```python
from build123d import *

# Parameters (mm, degrees)
SKETCH_1_R      = 25
SKETCH_1_R_2    = 2.1
EXTRUDE_1_DEPTH = 5
SKETCH_2_R      = 25
SKETCH_2_R_2    = 24
SKETCH_2_R_3    = 12
EXTRUDE_2_DEPTH = 4
FILLET_1_R      = 1
SKETCH_3_R      = 8
EXTRUDE_3_DEPTH = 15


with BuildPart() as part:
    # Эскиз1 → Бобышка-Вытянуть1 (new body)
    with BuildSketch(Plane(origin=(0, 0, 0), x_dir=(1, 0, 0), z_dir=(0, 1, 0))):
        with Locations(Location((0, 0, 0), (0, 0, 270))):
            Circle(SKETCH_1_R)
        with Locations(Location((-18, 0, 0), (0, 0, 270))):
            Circle(SKETCH_1_R_2, mode=Mode.SUBTRACT)
        with Locations(Location((-12.727922061, 12.727922061, 0), (0, 0, 270))):
            Circle(SKETCH_1_R_2, mode=Mode.SUBTRACT)
        with Locations(Location((0, 18, 0), (0, 0, 270))):
            Circle(SKETCH_1_R_2, mode=Mode.SUBTRACT)
        with Locations(Location((12.727922061, 12.727922061, 0), (0, 0, 270))):
            Circle(SKETCH_1_R_2, mode=Mode.SUBTRACT)
        with Locations(Location((18, 0, 0), (0, 0, 270))):
            Circle(SKETCH_1_R_2, mode=Mode.SUBTRACT)
        with Locations(Location((12.727922061, -12.727922061, 0), (0, 0, 270))):
            Circle(SKETCH_1_R_2, mode=Mode.SUBTRACT)
        with Locations(Location((0, -18, 0), (0, 0, 270))):
            Circle(SKETCH_1_R_2, mode=Mode.SUBTRACT)
        with Locations(Location((-12.727922061, -12.727922061, 0), (0, 0, 270))):
            Circle(SKETCH_1_R_2, mode=Mode.SUBTRACT)
    extrude(amount=EXTRUDE_1_DEPTH)

    # Эскиз2 → Бобышка-Вытянуть2 (add)
    # profile 1 of 10: a face of its own
    with BuildSketch(Plane(origin=(0, 5, 0), x_dir=(1, 0, 0), z_dir=(0, 1, 0))):
        with Locations(Location((0, 0, 0), (0, 0, 270))):
            Circle(SKETCH_2_R)
        Circle(SKETCH_2_R_2, mode=Mode.SUBTRACT)
    # profile 2 of 10: a face of its own
    with BuildSketch(Plane(origin=(0, 5, 0), x_dir=(1, 0, 0), z_dir=(0, 1, 0))):
        Circle(SKETCH_2_R_3)
    # profile 3 of 10: a face of its own
    with BuildSketch(Plane(origin=(0, 5, 0), x_dir=(1, 0, 0), z_dir=(0, 1, 0))):
        with BuildLine():
            Line((-10.332266323, 21.662046824), (-5.166133162, 10.831023412))
            ThreePointArc((-5.166133162, 10.831023412), (-4.592201188, 11.08655439), (-4.005682311, 11.311697893))
            Line((-4.005682311, 11.311697893), (-8.011364622, 22.623395786))
            ThreePointArc((-8.011364622, 22.623395786), (-9.184402377, 22.17310878), (-10.332266323, 21.662046824))
        make_face()
    # profile 4 of 10: a face of its own
    with BuildSketch(Plane(origin=(0, 5, 0), x_dir=(1, 0, 0), z_dir=(0, 1, 0))):
        with BuildLine():
            Line((8.011364622, 22.623395786), (4.005682311, 11.311697893))
            ThreePointArc((4.005682311, 11.311697893), (4.592201188, 11.08655439), (5.166133162, 10.831023412))
            Line((5.166133162, 10.831023412), (10.332266323, 21.662046824))
            ThreePointArc((10.332266323, 21.662046824), (9.184402377, 22.17310878), (8.011364622, 22.623395786))
        make_face()
    # profile 5 of 10: a face of its own
    with BuildSketch(Plane(origin=(0, 5, 0), x_dir=(1, 0, 0), z_dir=(0, 1, 0))):
        with BuildLine():
            ThreePointArc((10.831023412, 5.166133162), (11.08655439, 4.592201188), (11.311697893, 4.005682311))
            Line((11.311697893, 4.005682311), (22.623395786, 8.011364622))
            ThreePointArc((22.623395786, 8.011364622), (22.17310878, 9.184402377), (21.662046824, 10.332266323))
            Line((21.662046824, 10.332266323), (10.831023412, 5.166133162))
        make_face()
    # profile 6 of 10: a face of its own
    with BuildSketch(Plane(origin=(0, 5, 0), x_dir=(1, 0, 0), z_dir=(0, 1, 0))):
        with BuildLine():
            ThreePointArc((11.311697893, -4.005682311), (11.08655439, -4.592201188), (10.831023412, -5.166133162))
            Line((10.831023412, -5.166133162), (21.662046824, -10.332266323))
            ThreePointArc((21.662046824, -10.332266323), (22.17310878, -9.184402377), (22.623395786, -8.011364622))
            Line((22.623395786, -8.011364622), (11.311697893, -4.005682311))
        make_face()
    # profile 7 of 10: a face of its own
    with BuildSketch(Plane(origin=(0, 5, 0), x_dir=(1, 0, 0), z_dir=(0, 1, 0))):
        with BuildLine():
            ThreePointArc((5.166133162, -10.831023412), (4.592201188, -11.08655439), (4.005682311, -11.311697893))
            Line((4.005682311, -11.311697893), (8.011364622, -22.623395786))
            ThreePointArc((8.011364622, -22.623395786), (9.184402377, -22.17310878), (10.332266323, -21.662046824))
            Line((10.332266323, -21.662046824), (5.166133162, -10.831023412))
        make_face()
    # profile 8 of 10: a face of its own
    with BuildSketch(Plane(origin=(0, 5, 0), x_dir=(1, 0, 0), z_dir=(0, 1, 0))):
        with BuildLine():
            ThreePointArc((-4.005682311, -11.311697893), (-4.592201188, -11.08655439), (-5.166133162, -10.831023412))
            Line((-5.166133162, -10.831023412), (-10.332266323, -21.662046824))
            ThreePointArc((-10.332266323, -21.662046824), (-9.184402377, -22.17310878), (-8.011364622, -22.623395786))
            Line((-8.011364622, -22.623395786), (-4.005682311, -11.311697893))
        make_face()
    # profile 9 of 10: a face of its own
    with BuildSketch(Plane(origin=(0, 5, 0), x_dir=(1, 0, 0), z_dir=(0, 1, 0))):
        with BuildLine():
            Line((-21.662046824, -10.332266323), (-10.831023412, -5.166133162))
            ThreePointArc((-10.831023412, -5.166133162), (-11.08655439, -4.592201188), (-11.311697893, -4.005682311))
            Line((-11.311697893, -4.005682311), (-22.623395786, -8.011364622))
            ThreePointArc((-22.623395786, -8.011364622), (-22.17310878, -9.184402377), (-21.662046824, -10.332266323))
        make_face()
    # profile 10 of 10: a face of its own
    with BuildSketch(Plane(origin=(0, 5, 0), x_dir=(1, 0, 0), z_dir=(0, 1, 0))):
        with BuildLine():
            Line((-22.623395786, 8.011364622), (-11.311697893, 4.005682311))
            ThreePointArc((-11.311697893, 4.005682311), (-11.08655439, 4.592201188), (-10.831023412, 5.166133162))
            Line((-10.831023412, 5.166133162), (-21.662046824, 10.332266323))
            ThreePointArc((-21.662046824, 10.332266323), (-22.17310878, 9.184402377), (-22.623395786, 8.011364622))
        make_face()
    extrude(amount=EXTRUDE_2_DEPTH)

    # Скругление1
    fillet_1_edges = [part.edges().sort_by_distance(p)[0] for p in [
        (5.166133162, 7, 10.831023412),
        (10.831023412, 7, 5.166133162),
        (21.662046824, 7, 10.332266323),
        (22.623395786, 7, 8.011364622),
        (11.311697893, 7, 4.005682311),
        (11.311697893, 7, -4.005682311),
        (21.662046824, 7, -10.332266323),
        (10.831023412, 7, -5.166133162),
        (5.166133162, 7, -10.831023412),
        (8.011364622, 7, -22.623395786),
        (4.005682311, 7, -11.311697893),
        (-4.005682311, 7, -11.311697893),
        (-10.332266323, 7, -21.662046824),
        (-5.166133162, 7, -10.831023412),
        (-10.831023412, 7, -5.166133162),
        (-22.623395786, 7, -8.011364622),
        (-11.311697893, 7, -4.005682311),
        (-11.311697893, 7, 4.005682311),
        (-21.662046824, 7, 10.332266323),
        (-10.831023412, 7, 5.166133162),
        (-5.166133162, 7, 10.831023412),
        (-8.011364622, 7, 22.623395786),
        (-4.005682311, 7, 11.311697893),
        (4.005682311, 7, 11.311697893),
        (10.332266323, 7, 21.662046824),
        (22.623395786, 7, -8.011364622),
        (10.332266323, 7, -21.662046824),
        (-8.011364622, 7, -22.623395786),
        (-21.662046824, 7, -10.332266323),
        (-22.623395786, 7, 8.011364622),
        (-10.332266323, 7, 21.662046824),
        (8.011364622, 7, 22.623395786),
    ]]
    fillet(fillet_1_edges, radius=FILLET_1_R)

    # Эскиз3 → Бобышка-Вытянуть3 (add)
    with BuildSketch(Plane(origin=(0, 9, 0), x_dir=(1, 0, 0), z_dir=(0, 1, 0))):
        with Locations(Location((0, 0, 0), (0, 0, 270))):
            Circle(SKETCH_3_R)
    extrude(amount=EXTRUDE_3_DEPTH)


solid = part.part
```
The listing builds one solid part. Answer for the finished solid, in the listing's coordinates (mm). A direction names the side the tool comes from. Give positions to 0.01 mm unless a question says otherwise; leave off trailing zeros. Order: outer loops, then holes, each group sorted by start corner. A loop starts at its lowest first (then second) coordinate and runs counter-clockwise, first axis right, second up. Notation, with made-up numbers: M -12.75,89.25 L 3.25,89.25 A20 ccw 3.25,97.25 Z; hole C -11.5,58.25 d7. An arc over 180 degrees is marked long. Put each result on its own line as item: value. Start each with the question number.
Item 1: The part is cut by section D-D, the plane x = -18. Determine the outline of the cut face in (y, z), and give its area (3 significant figures).
Item 2: Flat-ended cylindrical pins translate along their axes: P1, Ø8, axis at x = -18.5, z = 6, coming from the -Y side; P2, Ø3.5, axis at x = 1, z = 18.5, coming from the +Y side; P3, Ø10, axis at x = -14, y = 8.5, coming from the -Z side; P4, Ø12.5, axis at x = 9.5, z = -13, coming from the +Y side. Find the tip coordinate at first contact, or state that the pin passes through.
Item 3: The part is cut by section B-B, the plane x = 0. Determine the outline of the cut face in (y, z).
Item 4: Find the intervals of material crossed by line 1 along X through (y, z) = (7.5, 0.5) (3 decimals); line 2 along X through (y, z) = (2.25, -13.5) (3 decimals); line 3 along Y through (x, z) = (20, -8), in increasing order.
Item 5: The part is cut by section A-A, the plane z = 0. Determine the outline of the cut face in (x, y), and give its area (3 significant figures).
Item 6: Which of the six approach directions +Z, -Z, +X, -X, +Y, -Y give full straight-line access (tool end or side, diameter ignored) to faces 1 (the face through (0, 0, 0)), 2 (the face through (7.616, 7.028, -22.454))?
Item 7: The part is cut by section C-C, the plane y = 2.75. State how many separate pieces and enclosed holes the cut face has, and give its area (3 significant figures).
Answer key:
1. outline: M 0,-17.35 L 9,-17.35 L 9,-15.87 L 5,-15.87 L 5,-8.59 L 9,-8.59 L 9,-6.37 L 5,-6.37 L 5,-2.1 L 0,-2.1 Z; M 0,2.1 L 5,2.1 L 5,6.37 L 9,6.37 L 9,8.59 L 5,8.59 L 5,15.87 L 9,15.87 L 9,17.35 L 0,17.35 Z
1. area: 182 mm²
2. P1: stops at y = 0
2. P2: stops at y = 5
2. P3: stops at z = -23.32
2. P4: stops at y = 9
3. outline: M 0,-25 L 9,-25 L 9,-24 L 5,-24 L 5,-20.1 L 0,-20.1 Z; M 0,-15.9 L 5,-15.9 L 5,-12 L 9,-12 L 9,-8 L 24,-8 L 24,8 L 9,8 L 9,12 L 5,12 L 5,15.9 L 0,15.9 Z; M 0,20.1 L 5,20.1 L 5,24 L 9,24 L 9,25 L 0,25 Z
4. line 1: x = -24.995 to -23.995, -11.99 to 11.99, 23.995 to 24.995
4. line 2: x = -21.042 to -14.681, -10.775 to 10.775, 14.681 to 21.042
4. line 3: y = 0 to 9
5. outline: M -25,0 L -20.1,0 L -20.1,5 L -24,5 L -24,9 L -25,9 Z; M -15.9,0 L 15.9,0 L 15.9,5 L 12,5 L 12,9 L 8,9 L 8,24 L -8,24 L -8,9 L -12,9 L -12,5 L -15.9,5 Z; M 20.1,0 L 25,0 L 25,9 L 24,9 L 24,5 L 20.1,5 Z
5. area: 552 mm²
6. face 1: +Z, -Z, +X, -X, -Y
6. face 2: +Y
7. separate pieces: 1
7. enclosed holes: 8
7. area: 1,850 mm²
